Check sheet for the drawn part. Datum: minimum x, y, z corner. Units: mm. Coordinates: 2 decimals unless noted, no trailing zeros. Write each loop counter-clockwise with the first axis right and the second up, starting at its lowest first coordinate (ties: lowest second). Pieces come first, ordered by that corner, then holes. Notation, with made-up numbers: (4, 31.25) -> (51, 31.25) arc R16 ccw to (51, 47.25) -> close; hole circle Ø10 at (0, -27). An arc over 180 degrees is marked (long way). Write item = value, one per line. Start each with the question number.
(1) Section check A-A (y = 14.9). Record the cut outline in (x, z).
(2) Gauge pin test, flat ends, axial feed: pin 1 Ø11 at (x, y) = (11, 19.5) entering from -Z; pin 2 Ø3 at (x, y) = (20, 14.9) entering from -Z. Record the tip position at first contact, or that the pin passes through.
(3) Section check D-D (x = 11). Record the cut outline in (y, z), plus the area to 3 significant figures.
(4) Material ranges on probe 1 along Y at (x, z) = (2, 2.4); probe 2 along X at (y, z) = (26, 2.1); probe 3 along Z at (x, y) = (5.5, 9.5), recorded low to high. Write a range as [from, to].
(5) Section check C-C (x = 20). Record the cut outline in (y, z).
(6) Section check B-B (z = 1.9). Record the cut outline in (x, y).
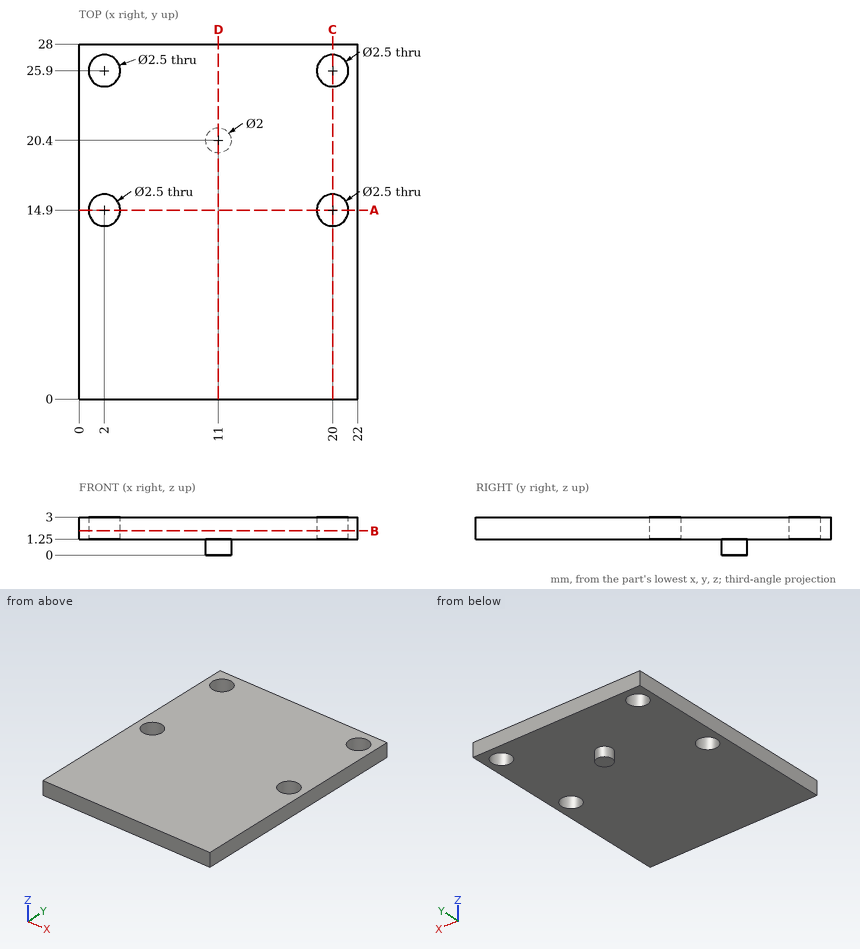
Response:
q1.outline = (0, 1.25) -> (0.75, 1.25) -> (0.75, 3) -> (0, 3) -> close; (3.25, 1.25) -> (18.75, 1.25) -> (18.75, 3) -> (3.25, 3) -> close; (21.25, 1.25) -> (22, 1.25) -> (22, 3) -> (21.25, 3) -> close
q2.pin_1 = 0
q2.pin_2 = 1.25
q3.outline = (0, 1.25) -> (19.4, 1.25) -> (19.4, 0) -> (21.4, 0) -> (21.4, 1.25) -> (28, 1.25) -> (28, 3) -> (0, 3) -> close
q3.area = 51.5 mm2
q4.probe_1 = [0, 13.65], [16.15, 24.65], [27.15, 28]
q4.probe_2 = [0, 0.75], [3.25, 18.75], [21.25, 22]
q4.probe_3 = [1.25, 3]
q5.outline = (0, 1.25) -> (13.65, 1.25) -> (13.65, 3) -> (0, 3) -> close; (16.15, 1.25) -> (24.65, 1.25) -> (24.65, 3) -> (16.15, 3) -> close; (27.15, 1.25) -> (28, 1.25) -> (28, 3) -> (27.15, 3) -> close
q6.outline = (0, 0) -> (22, 0) -> (22, 28) -> (0, 28) -> close; hole circle Ø2.5 at (2, 14.9); hole circle Ø2.5 at (2, 25.9); hole circle Ø2.5 at (20, 14.9); hole circle Ø2.5 at (20, 25.9)
